Autodesk Inventor part; units mm, degrees
ref_plane "YZ Plane" through (0, 0, 0) normal (1, 0, 0) x (0, 1, 0)
ref_plane "XZ Plane" through (0, 0, 0) normal (0, 1, 0) x (-1, 0, 0)
ref_plane "XY Plane" through (0, 0, 0) normal (0, 0, 1) x (1, 0, 0)
sketch "스케치1" plane through (0, 0, 0) normal (0, 1, 0) x (-1, 0, 0)
  circle A0 centre (0, 0) radius 2.85
  circle A1 centre (0, 0) radius 3.45
  dimension "d0" = 5.7
  dimension "d1" = 6.9
extrude "돌출1" add sketch "스케치1" along normal blind 2.5
sketch "스케치2" plane through (0, 2.5, 0) normal (0, 1, 0) x (1, 0, 0)
  circle A0 centre (0, 0) radius 3.45
  circle A1 centre (0, 0) radius 3.45
  line L0 (0.5, 3.4136) -> (-0.5, 3.4136)
  line L1 (-0.5, 3.4136) -> (-0.5, -3.4136)
  line L2 (-0.5, -3.4136) -> (0.5, -3.4136)
  line L3 (0.5, -3.4136) -> (0.5, 3.4136)
  line L4 (0.5, 3.4136) -> (-0.5, -3.4136) construction
  line L5 (-0.5, 3.4136) -> (0.5, -3.4136) construction
  point P0 (-0.5, -3.4136)
  point P1 (0.5, -3.4136)
  point P2 (0.5, 3.4136)
  point P3 (-0.5, 3.4136)
  dimension "d4" = 1
extrude "돌출2" add sketch "스케치2" along normal blind 2.4 contours L0 A0 | L3 L2 L1 L0 | A0 L2
chamfer "모따기1" distance 1 angle 45 4 edges at (0.5, 2.5, 3.1097) (0.5, 2.5, -3.1097) (-0.5, 2.5, -3.1097) (-0.5, 2.5, 3.1097)
chamfer "모따기2" distance 1 angle 45 4 edges at (-0.5, 3, -2.8058) (-0.5, 3, 2.8058) (0.5, 3, 2.8058) (0.5, 3, -2.8058)
properties part number "terminalcap_4.1mm_addon"
Input: part model. Units: mm. Frame: model coordinates. A direction names the side the tool comes from. Give positions to 0.01 mm unless a question says otherwise; leave off trailing zeros. Order: outer loops, then holes, each group sorted by start corner. A loop starts at its lowest first (then second) coordinate and runs counter-clockwise, first axis right, second up. Notation, with made-up numbers: (50, 15.25) - (108, 15.25) arc R27 cw to (108, 48.25) - close; hole circle Ø3 at (74, -21.75). An arc over 180 degrees is marked (long way). Write each question's results on one line, items separated by ' | '.
Item 1: Section A-A (z = 0). Return loops of the section in (x, y).
A:
outline: (-3.45, 0) - (-2.85, 0) - (-2.85, 2.5) - (-3.45, 2.5) - close; (-0.5, 2.5) - (0.5, 2.5) - (0.5, 4.9) - (-0.5, 4.9) - close; (2.85, 0) - (3.45, 0) - (3.45, 2.5) - (2.85, 2.5) - close
Item 2: Material intervals for line 1 along Z through (x, y) = (0, 1.85); line 2 along Y through (x, z) = (0.25, 0); line 3 along Y through (x, z) = (-3, 0), sorted ascending.
A:
line 1: z = -3.45 to -2.85, 2.85 to 3.45 | line 2: y = 2.5 to 4.9 | line 3: y = 0 to 2.5
Item 3: Section C-C (x = 0). Return loops of the section in (y, z).
A:
outline: (0, -3.45) - (4.9, -3.45) - (4.9, 3.45) - (0, 3.45) - (0, 2.85) - (2.5, 2.85) - (2.5, -2.85) - (0, -2.85) - close
Item 4: Section B-B (x = -2.75). Return loops of the section in (y, z).
A:
outline: (0, -2.08) - (2.5, -2.08) - (2.5, -0.75) - (0, -0.75) - close; (0, 0.75) - (2.5, 0.75) - (2.5, 2.08) - (0, 2.08) - close
Item 5: Draft query along X for faces 1 (the flat face through (0, 2.5, 0)), 2 (the flat face through (1, 3, 3)), 3 (the flat face through (-1, 3, 3)). Return one class per face: released by +X, released by -X, zero draft, split by the parting line, or undercut.
A:
face 1: undercut | face 2: released by +X | face 3: released by -X
Item 6: Contact query for flat-ended pins moving along their axis: pin 1 Ø1.6 at (x, z) = (-3, -1.5) entering from +Y; pin 2 Ø2 at (x, y) = (-2, 2) entering from +Z; pin 3 Ø1.9 at (y, z) = (3.5, 0) entering from -X. Output: stop coordinate, or through.
A:
pin 1: stops at y = 2.5 | pin 2: stops at z = 3.3 | pin 3: stops at x = -0.5
Item 7: Section D-D (z = -0.75). Return loops of the section in (x, y).
A:
outline: (-3.37, 0) - (-2.75, 0) - (-2.75, 2.5) - (-3.37, 2.5) - close; (-0.5, 2.5) - (0.5, 2.5) - (0.5, 4.9) - (-0.5, 4.9) - close; (2.75, 0) - (3.37, 0) - (3.37, 2.5) - (2.75, 2.5) - close
Item 8: Access query for faces 4 (the flat face through (3.1, 2.5, 0.2)), 5 (the flat face through (-0.5, 4, 0)), 6 (the cylindrical face through (2.262, 1.263, 1.734)), 7 (the flat face through (0.5, 4, 0)), 8 (the flat face through (-3, 2.5, -0.2)). Directions: +Z, -Z, +X, -X, +Y, -Y. A direction counts if a zero-diameter tool reaches every point of the face in a straight line with its end or side. Return the directions, or none.
A:
face 4: +Z, -Z, +X, +Y | face 5: -X, +Y | face 6: -Y | face 7: +X, +Y | face 8: +Z, -Z, -X, +Y
